Source: CAD feature listing. Evaluate the final solid. Frame: model axes, mm. A direction names the side the tool comes from. Give positions to 0.01 mm unless a question says otherwise; leave off trailing zeros. Write each loop counter-clockwise with the first axis right and the second up, starting at its lowest first coordinate (ties: lowest second). Pieces come first, ordered by that corner, then holes.
```python
from build123d import *

# Parameters (mm, degrees)
F0_R     = 29
F1_DEPTH = 1.6
F0_R_2   = 30.6
F2_DEPTH = 35
F5_R     = 10
F6_DEPTH = 40


with BuildPart() as f1:
    # F0 (on Top) → F1 (new body)
    with BuildSketch(Plane.XY):
        Circle(F0_R)
    extrude(amount=F1_DEPTH)

    # F0 (on Top) → F2 (join)
    with BuildSketch(Plane.XY):
        Circle(F0_R_2)
        Circle(F0_R, mode=Mode.SUBTRACT)
    extrude(amount=F2_DEPTH)

    # F4: sweep along a path in F4_path
    with BuildLine(Plane(origin=(30.6, 0, 35), x_dir=(0, 1, 0), z_dir=(0, 0, 1))) as f4_path:
        CenterArc((0, 30.6), 30.6, 0, 360)
    # F3 (on Front) → F4 (sweep)
    with BuildSketch(Plane.XZ):
        with BuildLine():
            Line((-33.2449047106, 50), (-31.3596123494, 39.3079757071))
            ThreePointArc((-31.3596123494, 39.3079757071), (-30.7902650954, 34.9833539611), (-30.6, 30.6255668237))
            Line((-30.6, 30.6255668237), (-30.6, 35))
            Line((-30.6, 35), (-29, 35))
            Line((-29, 35), (-31.6449047106, 50))
            Line((-31.6449047106, 50), (-33.2449047106, 50))
        make_face()
    sweep(path=f4_path.line)

    # F5 (on Right) → F6 (cut, symmetric)
    with BuildSketch(Plane.YZ):
        with Locations((0, 55)):
            Circle(F5_R)
    extrude(amount=F6_DEPTH, both=True, mode=Mode.SUBTRACT)


solid = f1.part
```
1. Line query: probe 1 along X at (y, z) = (0, 24); probe 2 along Z at (x, y) = (-19, -0.5). Output: solid intervals per line, ascending.
2. Section query B-B (z = 29.5). Return loops of the section in (x, y), plus the area to 3 significant figures.
3. Section query A-A (y = 0). Return loops of the section in (x, z).
4. Pin query (flat end, axial travel): P1, Ø3, axis at y = 16.5, z = 27.5, coming from the +X side; P2, Ø4, axis at x = -1, z = 24, coming from the -Y side; P3, Ø10, axis at x = 18, z = 12, coming from the +Y side. Return the tip coordinate at first contact, or that it passes through.
5. Access query for faces 4 (the cylindrical face through (13.38, -25.73, 18.07)), 5 (the conical face through (27.903, 14.513, 39.827)). Directions: +Z, -Z, +X, -X, +Y, -Y. A direction counts if a zero-diameter tool reaches every point of the face in a straight line with its end or side. Return the directions, or none.
6. Pull-direction query (X, two-part tool) for faces 1 (the flat face through (0, 0, 1.6)), 2 (the flat face through (0, 0, 0)), 3 (the cylindrical face through (29.187, 9.191, 15.098)); classes: pulls with the +X half, pulls with the -X half, needs draft (parallel to the pull), parting line crosses it, or undercut.
The answers:
1. probe 1: x = -30.6 to -29, 29 to 30.6
1. probe 2: z = 0 to 1.6
2. outline: circle Ø61.2 at (0, 0); hole circle Ø58 at (0, 0)
2. area: 300 mm2
3. outline: (-32.36, 45) - (-31.36, 39.31) arc R50 cw to (-30.6, 30.63) - (-30.6, 0) - (30.6, 0) - (30.6, 30.63) arc R50 cw to (31.36, 39.31) - (32.36, 45) - (30.76, 45) - (29, 35) - (29, 1.6) - (-29, 1.6) - (-29, 35) - (-30.76, 45) - close
4. P1: stops at x = 26.67
4. P2: stops at y = -30.6
4. P3: stops at y = 27.7
5. face 4: +Z
5. face 5: -Z
6. face 1: undercut
6. face 2: needs draft
6. face 3: parting line crosses it
